Work out the finished part from the listing and answer in its coordinate system (mm). Round coordinates to 2 decimals unless told otherwise and drop trailing zeros. Loops run counter-clockwise (first coordinate to the right, second up) from the corner with the lowest first, then second, coordinate; pieces in that order, holes last. Notation, with made-up numbers: (-39, -23.5) - (-9, -23.5) arc R29 cw to (-9, 15.5) - close; hole circle Ø11 at (67.5, -16.5). An arc over 180 degrees is marked (long way). Return JSON: item names as keys, results as strings.
from build123d import *

# Parameters (mm, degrees)
F1_ANGLE = -60


with BuildPart() as f1:
    # F0 (on Front) → F1 (revolve)
    with BuildSketch(Plane.XZ):
        with BuildLine():
            Line((-50, 20.325956), (-50, -19.674044))
            Line((-50, -19.674044), (0, -19.674044))
            Line((0, -19.674044), (50, -19.674044))
            Line((50, -19.674044), (50, 20.325956))
            Line((50, 20.325956), (35, 20.325956))
            ThreePointArc((35, 20.325956), (0, -14.674044), (-35, 20.325956))
            Line((-35, 20.325956), (-50, 20.325956))
        make_face()
    revolve(axis=Axis((-60, 0, 1.129986), (0, 0, -1)), revolution_arc=F1_ANGLE)


solid = f1.part
1) Flat-ended cylindrical pins translate along their axes: pin 1 (6 mm diameter, centred on x = 7.5, z = -13.5, fed in from +Y); pin 2 (12 mm diameter, centred on x = -44, z = -15.5, fed in from +Y); pin 3 (8 mm diameter, centred on y = 85.5, z = -2, fed in from +X); pin 4 (12 mm diameter, centred on x = -39.5, y = 48.5, fed in from +Z). Find the tip coordinate at first contact, or state that the pin passes through.
Verdict:
{"pin 1": "stops at y = 89.11", "pin 2": "stops at y = 38.11", "pin 3": "stops at x = 13.88", "pin 4": "passes through"}
2) Section B-B (z = 5.5) is taken. Give the vertices of the cut face in (x, y), and give its area (3 significant figures).
Verdict:
{"outline": "(-55, 8.66) arc R10 cw to (-50, 0) - (-31.7, 0) arc R28.3 ccw to (-45.85, 24.5) - close; (-14.15, 79.42) arc R91.7 cw to (31.7, 0) - (50, 0) arc R110 ccw to (-5, 95.26) - close", "area": "2,300 mm2"}
3) Find the intervals of material crossed by L1, parallel to X at y = 17, z = 8; L2, parallel to X at y = 17.5, z = -3.5; L3, parallel to X at y = 78, z = -7.5, in increasing order.
Verdict:
{"L1": "x = -50.19 to -38.71, 31.19 to 48.68", "L2": "x = -49.9 to -30.43, 23.83 to 48.6", "L3": "x = -14.97 to 17.56"}
4) Section C-C (x = 41) is taken. Give the vertices of the cut face in (y, z), and give its area (3 significant figures).
Verdict:
{"outline": "(0, -19.67) - (43.58, -19.67) - (43.58, 20.33) - (0, 20.33) - close", "area": "1,740 mm2"}
5) Section A-A (z = -7.5) is taken. Give the vertices of the cut face in (x, y).
Verdict:
{"outline": "(-55, 8.66) arc R10 cw to (-50, 0) - (-21.23, 0) arc R38.77 ccw to (-40.62, 33.58) - close; (-19.38, 70.35) arc R81.23 cw to (21.23, 0) - (50, 0) arc R110 ccw to (-5, 95.26) - close"}
6) Section D-D (y = 89.5) is taken. Give the vertices of the cut face in (x, z).
Verdict:
{"outline": "(-8.33, -19.67) - (3.95, -19.67) - (3.95, 20.33) - (-8.33, 20.33) - close"}
